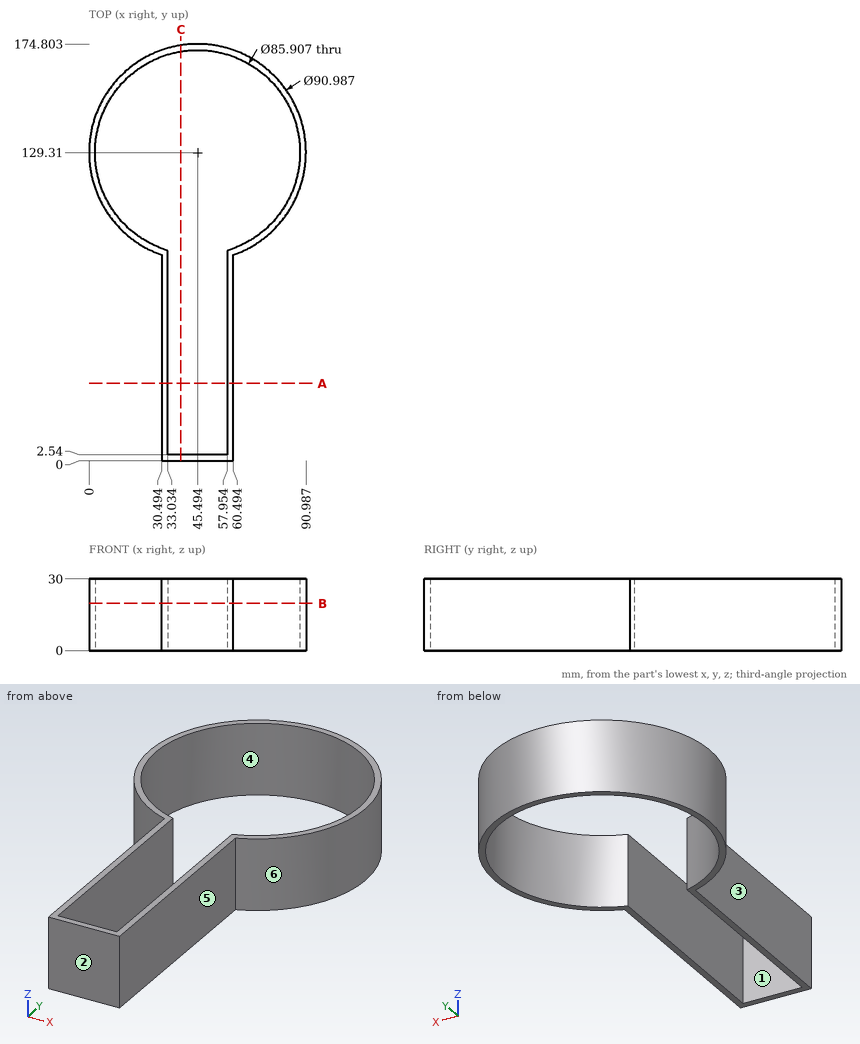
Geometry check sheet. Reference: drawing and pictorial views, mm from the part's lowest x, y, z. A direction names the side the tool comes from. Give positions to 0.01 mm unless a question says otherwise; leave off trailing zeros. Order: outer loops, then holes, each group sorted by start corner. A loop starts at its lowest first (then second) coordinate and runs counter-clockwise, first axis right, second up. Notation, with made-up numbers: M 86,-27.75 L 118,-27.75 A25 cw 118,-6.75 Z; hole C 85,61 d4. An arc over 180 degrees is marked long. Answer in a Markdown table with one row per item. Add a question column.
Q1. Access from +Z, -Z, +X, -X, +Y, -Y to the whole of each face (thin tool, end or side, straight path). Record for the marked faces 1, 2 and 3.
Q2. Gauge pin test, flat ends, axial feed: pin 1 Ø4 at (y, z) = (75.5, 27) entering from +X; pin 2 Ø1.5 at (x, z) = (24.5, 22) entering from +Y; pin 3 Ø1.5 at (x, y) = (57, 84) entering from -Z; pin 4 Ø2 at (x, z) = (79, 4) entering from +Y. Record the tip position at first contact, or that the pin passes through.
Q3. Thickness scan on L1, parallel to X at y = 13, z = 17; L2, parallel to X at y = 129, z = 12.5; L3, parallel to Y at x = 63.5, z = 23.5. Record the ranges inside material, lowest first.
Q4. Release check for a two-part mould opening along Y. For the marked faces 4, 5 and 6 record: released by +Y, released by -Y, zero draft, split by the parting line, or undercut.
Q5. Sectioned sample at C-C, the plane x = 38.5. Record the boundary of the cut face in (y, z).
Q6. Sectioned sample at B-B, the plane z = 19.75. Record the boundary of the cut face in (x, y), and give its area (3 significant figures).
Q7. Sectioned sample at A-A, the plane y = 32.5. Record the boundary of the cut face in (x, z).
Verdict:
| question | item | result |
|---|---|---|
| 1 | face 1 | +Z, -Z |
| 1 | face 2 | +Z, -Z, +X, -X, -Y |
| 1 | face 3 | +Z, -Z, -X, -Y |
| 2 | pin 1 | x = 60.49 |
| 2 | pin 2 | y = 170.05 |
| 2 | pin 3 | through |
| 2 | pin 4 | y = 161.14 |
| 3 | L1 | 30.49 to 33.03, 57.95 to 60.49 |
| 3 | L2 | 0 to 2.54, 88.45 to 90.99 |
| 3 | L3 | 87.53 to 90.31, 168.31 to 171.09 |
| 4 | face 4 | undercut |
| 4 | face 5 | zero draft |
| 4 | face 6 | split by the parting line |
| 5 | outline | M 0,0 L 2.54,0 L 2.54,30 L 0,30 Z; M 171.69,0 L 174.26,0 L 174.26,30 L 171.69,30 Z |
| 6 | outline | M 30.49,0 L 60.49,0 L 60.49,86.36 A45.49 ccw long 30.49,86.36 Z; hole M 33.03,2.54 L 57.95,2.54 L 57.95,88.2 A42.95 ccw long 33.03,88.2 Z |
| 6 | area | 1,140 mm² |
| 7 | outline | M 30.49,0 L 33.03,0 L 33.03,30 L 30.49,30 Z; M 57.95,0 L 60.49,0 L 60.49,30 L 57.95,30 Z |
